```python
from build123d import *

# Parameters (mm, degrees)
F4_R     = 37.2842712475
F4_R_2   = 32.2842712475
F5_DEPTH = 12.5
F6_R     = 1.5


# Not quite as in the source:
# - a pattern or mirror of a feature is missing from the dataset's text; its kind, count and spacing are read off the source's solid


with BuildPart() as f1:
    # F0 (on Front) → F1 (revolve)
    with BuildSketch(Plane.XZ):
        with BuildLine():
            Line((32.2842712475, 10), (28.2842712475, 10))
            ThreePointArc((28.2842712475, 10), (30, 0), (28.2842712475, -10))
            Line((28.2842712475, -10), (32.2842712475, -10))
            Line((32.2842712475, -10), (32.2842712475, 10))
        make_face()
    revolve(axis=Axis((0, 0, -0.0082536135), (0, 0, -1)))

    # F2 (on Right) → F3 (revolve)
    with BuildSketch(Plane.YZ):
        Polygon((-21.5096189432, 0), (-34.5, 7.5), (-34.5, 0), align=None)
    f3 = revolve(axis=Axis((0, -28.0048094716, 0), (0, -1, 0)))

    # F3_copies: F3 across plane
    add(f3.mirror(Plane.ZX))

    # F4 (on Top) → F5 (cut, symmetric)
    with BuildSketch(Plane.XY):
        Circle(F4_R)
        Circle(F4_R_2, mode=Mode.SUBTRACT)
    extrude(amount=F5_DEPTH, both=True, mode=Mode.SUBTRACT)

    # F6
    f6_edges = [f1.edges().sort_by_distance(p)[0] for p in [
        (-32.284271, 0, 10),
        (-32.284271, 0, -10),
    ]]
    fillet(f6_edges, radius=F6_R)


solid = f1.part
```
CAD build for the part. Positions are in the model's coordinates, mm. Round coordinates to 2 decimals unless told otherwise and drop trailing zeros. Write each loop counter-clockwise with the first axis right and the second up, starting at its lowest first coordinate (ties: lowest second). Pieces come first, ordered by that corner, then holes. Notation, with made-up numbers: (53.5, -24.75) - (80.5, -24.75) arc R12 cw to (80.5, -11.75) - close; hole circle Ø6 at (-26, 50.5). An arc over 180 degrees is marked (long way). Write item = value, one per line. Start each with the question number.
Q1. Mould opens along Z. For faces 1 (the flat face through (-14, 25, -10)), 2 (the flat face through (14, 25, 10)), 3 (the conical face through (1.13, 24.72, -1.47)) say: pulls with the +Z half, pulls with the -Z half, needs draft (parallel to the pull), parting line crosses it, or undercut.
Q2. Band-saw the part on B-B (z = 7.5). Give the cut face in (x, y), then the cut area to 3 significant figures.
Q3. Probe L1, parallel to Y at x = -21.5, z = 5.75; L2, parallel to X at y = -18, z = -0.75; L3, parallel to X at y = 22.5, z = 5. List the from-to ranges inside material, lowest first. Write a range as from..to.
Q4. Band-saw the part on A-A (y = 0). Give the cut face in (x, z).
Q5. Drop flat-ended pins along their axis: pin 1 (4 mm diameter, centred on x = -18, z = 1.5, fed in from -Y); pin 2 (10 mm diameter, centred on y = -13.5, z = -4, fed in from +X); pin 3 (12 mm diameter, centred on x = -8.5, z = 0, fed in from -Y). Give the stop position or say it passes through.
Answers below:
q1.face_1 = pulls with the -Z half
q1.face_2 = pulls with the +Z half
q1.face_3 = undercut
q2.outline = circle Ø64.57 at (0, 0); hole circle Ø58.09 at (0, 0)
q2.area = 624 mm2
q3.L1 = -24.08..-20.12, 20.12..24.08
q3.L2 = -26.8..-23.99, 23.99..26.8
q3.L3 = -23.15..-19.2, 19.2..23.15
q4.outline = (-32.28, -8.5) arc R1.5 ccw to (-30.78, -10) - (-28.28, -10) arc R30 cw to (-28.28, 10) - (-30.78, 10) arc R1.5 ccw to (-32.28, 8.5) - close; (28.28, -10) - (30.78, -10) arc R1.5 ccw to (32.28, -8.5) - (32.28, 8.5) arc R1.5 ccw to (30.78, 10) - (28.28, 10) arc R30 cw to start
q5.pin_1 = -28.04
q5.pin_2 = 31.15
q5.pin_3 = -32.19
